from build123d import *

# Parameters (mm, degrees)
SKETCH1_R           = 7.5
BOSS_EXTRUDE1_DEPTH = 13
SKETCH2_R           = 6.5
CUT_EXTRUDE1_DEPTH  = 7
SKETCH3_W           = 8
SKETCH3_H           = 5
CUT_EXTRUDE2_DEPTH  = 5
SKETCH5_R           = 5
CUT_EXTRUDE5_DEPTH  = 5
SKETCH7_R           = 0.9
BOSS_EXTRUDE4_DEPTH = 14
SKETCH10_R          = 2
BOSS_EXTRUDE5_DEPTH = 5
BOSS_EXTRUDE6_START = -5
SKETCH11_R          = 2
BOSS_EXTRUDE6_DEPTH = 5
SKETCH13_R          = 7.5
CUT_EXTRUDE6_DEPTH  = 2
CHAMFER1_SIZE       = 1


with BuildPart() as part:
    # Sketch1 → Boss-Extrude1 (new body)
    with BuildSketch(Plane(origin=(0, 0, 0), x_dir=(1, 0, 0), z_dir=(0, 1, 0))):
        with Locations(Location((0, 0, 0), (0, 0, 90))):
            Circle(SKETCH1_R)
    extrude(amount=BOSS_EXTRUDE1_DEPTH)

    # Sketch2 → Cut-Extrude1 (cut)
    with BuildSketch(Plane.XZ):
        with Locations(Location((0, 0, 0), (0, 0, 270))):
            Circle(SKETCH2_R)
    extrude(amount=-CUT_EXTRUDE1_DEPTH, mode=Mode.SUBTRACT)

    # Sketch3 → Cut-Extrude2 (cut)
    with BuildSketch(Plane.XZ.offset(-7)):
        Rectangle(SKETCH3_W, SKETCH3_H)
    extrude(amount=-CUT_EXTRUDE2_DEPTH, mode=Mode.SUBTRACT)

    # Sketch5 → Cut-Extrude5 (cut)
    with BuildSketch(Plane.XZ.offset(-7)):
        with Locations(Location((0, 0, 0), (0, 0, 270))):
            Circle(SKETCH5_R)
    extrude(amount=-CUT_EXTRUDE5_DEPTH, mode=Mode.SUBTRACT)

    # Sketch7 → Boss-Extrude4 (add)
    with BuildSketch(Plane.XY.offset(7)):
        with Locations((0, 8)):
            Circle(SKETCH7_R)
    extrude(amount=-BOSS_EXTRUDE4_DEPTH)

    # Sketch10 → Boss-Extrude5 (add)
    with BuildSketch(Plane.XY.offset(2)):
        with Locations(Location((0, 8, 0), (0, 0, 209.999999411))):
            Circle(SKETCH10_R)
    extrude(amount=BOSS_EXTRUDE5_DEPTH)

    # Sketch11 → Boss-Extrude6 (add)
    with BuildSketch(Plane.XY.offset(-2).offset(BOSS_EXTRUDE6_START)):
        with Locations(Location((0, 8, 0), (0, 0, 209.999999411))):
            Circle(SKETCH11_R)
    extrude(amount=BOSS_EXTRUDE6_DEPTH)

    # Sketch13 → Cut-Extrude6 (cut)
    with BuildSketch(Plane.XZ):
        with Locations(Location((0, 0, 0), (0, 0, 270))):
            Circle(SKETCH13_R)
    extrude(amount=-CUT_EXTRUDE6_DEPTH, mode=Mode.SUBTRACT)

    # Chamfer1
    chamfer1_edges = [part.edges().sort_by_distance(p)[0] for p in [
        (0, 2, 6.5),
    ]]
    chamfer(chamfer1_edges, length=CHAMFER1_SIZE - 0.0001)  # a hair under: the kernel refuses the full size


solid = part.part
Input: part model. Units: mm. Frame: model coordinates. A direction names the side the tool comes from. Coordinates: 2 decimals unless noted, no trailing zeros. Loops run counter-clockwise (first coordinate to the right, second up) from the corner with the lowest first, then second, coordinate; pieces in that order, holes last. Notation, with made-up numbers: (73, 25.5) - (119, 25.5) arc R22 ccw to (119, 62.5) - close; hole circle Ø6 at (89.5, 55). An arc over 180 degrees is marked (long way). Answer in a Markdown table with one row per item. Add a question column.
Item 1: Section query D-D on y = 5.25. Return the cut outline in (x, z).
Item 2: Mould query, pull axis Y, two halves, no side actions, for faces 3 (the flat face through (0, 13, 0)), 4 (the flat face through (5.2, 7, 0.1)), 5 (the flat face through (0, 12, 0)), 6 (the cylindrical face through (-0.33, 7.423, 7.493)). Classes: released by +Y, released by -Y, zero draft, split by the parting line, or undercut.
Item 3: Access query for faces 1 (the flat face through (-5.2, 7, -0.4)), 2 (the cylindrical face through (0, 6, -4)). Directions: +Z, -Z, +X, -X, +Y, -Y. A direction counts if a zero-diameter tool reaches every point of the face in a straight line with its end or side. Return the directions, or none.
Item 4: Contact query for flat-ended pins moving along their axis: P1, Ø5, axis at x = 0.5, z = 1.5, coming from the -Y side; P2, Ø1, axis at x = -5.5, y = 3.5, coming from the +Z side; P3, Ø1, axis at x = 2.5, y = 11.5, coming from the +Z side. Output: stop coordinate, or through.
Item 5: Section query C-C on y = 7.5. Return the cut outline in (x, z), then the cut area to 3 significant figures.
Item 6: Line query: line 1 along Z through (x, y) = (0, 9.05); line 2 along X through (y, z) = (4.25, 0). Output: solid intervals per line, ascending. Write a range as [from, to].
Recorded:
| question | item | result |
|---|---|---|
| 1 | outline | circle Ø15 at (0, 0); hole circle Ø13 at (0, 0) |
| 2 | face 3 | released by +Y |
| 2 | face 4 | released by -Y |
| 2 | face 5 | undercut |
| 2 | face 6 | zero draft |
| 3 | face 1 | -Y |
| 3 | face 2 | none |
| 4 | P1 | y = 6 |
| 4 | P2 | z = 5.59 |
| 4 | P3 | z = 7.23 |
| 5 | outline | circle Ø15 at (0, 0); hole (-1.94, -4.61) - (-1.94, -2) - (-0.75, -2) - (-0.75, 2) - (-1.94, 2) - (-1.94, 4.61) arc R5 ccw to start; hole (0.75, -2) - (1.94, -2) - (1.94, -4.61) arc R5 ccw to (1.94, 4.61) - (1.94, 2) - (0.75, 2) - close |
| 5 | area | 126 mm^2 |
| 6 | line 1 | [-7.5, -2], [2, 7.5] |
| 6 | line 2 | [-7.5, -6.5], [6.5, 7.5] |
